from build123d import *

# Parameters (mm, degrees)
SKETCH_1_R          = 13
EXTRUDE_2_DEPTH     = 10
CUT_EXTRUDE_1_DEPTH = 21.928449536
SKETCH_3_R          = 7.5
CUT_EXTRUDE_2_DEPTH = 4
CUT_EXTRUDE_2_DRAFT = 6
SKETCH_4_R          = 7.5
CUT_EXTRUDE_3_DEPTH = 4
CUT_EXTRUDE_3_DRAFT = 6
SKETCH_5_R          = 4
EXTRUDE_3_DEPTH     = 30
CHAMFER_1_SIZE      = 1


with BuildPart() as part:
    # Эскиз1 → Бобышка-Вытянуть2 (new body)
    with BuildSketch(Plane.XY):
        Circle(SKETCH_1_R)
    extrude(amount=-EXTRUDE_2_DEPTH)

    # Эскиз2 → Вырез-Вытянуть1 (cut, through all)
    with BuildSketch(Plane.XY):
        with BuildLine():
            ThreePointArc((1.252557909, 8.912412619), (0, 9), (-1.252557909, 8.912412619))
            ThreePointArc((-1.252557909, 8.912412619), (-1.684886314, 10.969320472), (-2.924363706, 12.666810842))
            ThreePointArc((-2.924363706, 12.666810842), (0, 13), (2.924363706, 12.666810842))
            ThreePointArc((2.924363706, 12.666810842), (1.684886314, 10.969320472), (1.252557909, 8.912412619))
        make_face()
        with BuildLine():
            ThreePointArc((9.308326268, 9.074968986), (7.028330627, 10.936295927), (4.388063669, 12.237029756))
            ThreePointArc((4.388063669, 12.237029756), (4.513045823, 10.138897913), (3.764695278, 8.174782533))
            ThreePointArc((3.764695278, 8.174782533), (4.865767357, 7.571281795), (5.872132809, 6.82041467))
            ThreePointArc((5.872132809, 6.82041467), (7.34787895, 8.317061286), (9.308326268, 9.074968986))
        make_face()
        with BuildLine():
            ThreePointArc((12.736961008, 2.601888597), (11.82521594, 5.400395169), (10.307311834, 7.922078184))
            ThreePointArc((10.307311834, 7.922078184), (9.278117798, 6.089446906), (7.586684314, 4.841716754))
            ThreePointArc((7.586684314, 4.841716754), (8.186687958, 3.738735117), (8.627347034, 2.562983254))
            ThreePointArc((8.627347034, 2.562983254), (10.677971938, 3.024193907), (12.736961008, 2.601888597))
        make_face()
        with BuildLine():
            ThreePointArc((12.121700624, -4.697273037), (12.867678744, -1.850092898), (12.95406132, 1.091922764))
            ThreePointArc((12.95406132, 1.091922764), (11.097452929, 0.106639531), (8.999954685, -0.028559885))
            ThreePointArc((8.999954685, -0.028559885), (8.908392977, -1.280833544), (8.643439533, -2.508177236))
            ThreePointArc((8.643439533, -2.508177236), (10.617884283, -3.228833669), (12.121700624, -4.697273037))
        make_face()
        with BuildLine():
            ThreePointArc((7.657885939, -10.505083671), (9.824744467, -8.513189541), (11.487987866, -6.084910418))
            ThreePointArc((11.487987866, -6.084910418), (9.393425165, -5.910025141), (7.555803034, -4.889768962))
            ThreePointArc((7.555803034, -4.889768962), (6.801746169, -5.893746606), (5.915301052, -6.783009175))
            ThreePointArc((5.915301052, -6.783009175), (7.186693389, -8.456729369), (7.657885939, -10.505083671))
        make_face()
        with BuildLine():
            ThreePointArc((0.762746577, -12.977604465), (3.662523239, -12.473408657), (6.374559434, -11.329827537))
            ThreePointArc((6.374559434, -11.329827537), (4.707051283, -10.050298589), (3.712737307, -8.198510943))
            ThreePointArc((3.712737307, -8.198510943), (2.535593012, -8.635436763), (1.309096282, -8.904283628))
            ThreePointArc((1.309096282, -8.904283628), (1.473778124, -10.999673247), (0.762746577, -12.977604465))
        make_face()
        with BuildLine():
            ThreePointArc((-6.374559434, -11.329827537), (-3.662523239, -12.473408657), (-0.762746577, -12.977604465))
            ThreePointArc((-0.762746577, -12.977604465), (-1.473778124, -10.999673247), (-1.309096282, -8.904283628))
            ThreePointArc((-1.309096282, -8.904283628), (-2.535593012, -8.635436763), (-3.712737307, -8.198510943))
            ThreePointArc((-3.712737307, -8.198510943), (-4.707051283, -10.050298589), (-6.374559434, -11.329827537))
        make_face()
        with BuildLine():
            ThreePointArc((-11.487987866, -6.084910418), (-9.824744467, -8.513189541), (-7.657885939, -10.505083671))
            ThreePointArc((-7.657885939, -10.505083671), (-7.186693389, -8.456729369), (-5.915301052, -6.783009175))
            ThreePointArc((-5.915301052, -6.783009175), (-6.801746169, -5.893746606), (-7.555803034, -4.889768962))
            ThreePointArc((-7.555803034, -4.889768962), (-9.393425165, -5.910025141), (-11.487987866, -6.084910418))
        make_face()
        with BuildLine():
            ThreePointArc((-12.95406132, 1.091922764), (-12.867678744, -1.850092898), (-12.121700624, -4.697273037))
            ThreePointArc((-12.121700624, -4.697273037), (-10.617884283, -3.228833669), (-8.643439533, -2.508177236))
            ThreePointArc((-8.643439533, -2.508177236), (-8.908392977, -1.280833544), (-8.999954685, -0.028559885))
            ThreePointArc((-8.999954685, -0.028559885), (-11.097452929, 0.106639531), (-12.95406132, 1.091922764))
        make_face()
        with BuildLine():
            ThreePointArc((-10.307311834, 7.922078184), (-11.82521594, 5.400395169), (-12.736961008, 2.601888597))
            ThreePointArc((-12.736961008, 2.601888597), (-10.677971938, 3.024193907), (-8.627347034, 2.562983254))
            ThreePointArc((-8.627347034, 2.562983254), (-8.186687958, 3.738735117), (-7.586684314, 4.841716754))
            ThreePointArc((-7.586684314, 4.841716754), (-9.278117798, 6.089446906), (-10.307311834, 7.922078184))
        make_face()
        with BuildLine():
            ThreePointArc((-4.388063669, 12.237029756), (-7.028330627, 10.936295927), (-9.308326268, 9.074968986))
            ThreePointArc((-9.308326268, 9.074968986), (-7.34787895, 8.317061286), (-5.872132809, 6.82041467))
            ThreePointArc((-5.872132809, 6.82041467), (-4.865767357, 7.571281795), (-3.764695278, 8.174782533))
            ThreePointArc((-3.764695278, 8.174782533), (-4.513045823, 10.138897913), (-4.388063669, 12.237029756))
        make_face()
    extrude(amount=-CUT_EXTRUDE_1_DEPTH, mode=Mode.SUBTRACT)


with BuildPart() as cut_extrude_2_tool:
    # Эскиз3 → Вырез-Вытянуть2 (with draft: the straight prism first)
    with BuildSketch(Plane.XY):
        Circle(SKETCH_3_R)
    extrude(amount=-CUT_EXTRUDE_2_DEPTH)
    # Вырез-Вытянуть2: the draft: its side faces are tilted about the plane it starts from
    cut_extrude_2_sides = [cut_extrude_2_tool.faces().sort_by_distance(p)[0] for p in [
        (-7.5, 0, -2),
    ]]
    draft(cut_extrude_2_sides, Plane.XY, CUT_EXTRUDE_2_DRAFT)


with BuildPart() as part_1:
    add(part.part)

    # Вырез-Вытянуть2: cut by cut_extrude_2_tool
    add(cut_extrude_2_tool.part, mode=Mode.SUBTRACT)


with BuildPart() as cut_extrude_3_tool:
    # Эскиз4 → Вырез-Вытянуть3 (with draft: the straight prism first)
    with BuildSketch(Plane(origin=(0, 0, -10), x_dir=(-1, 0, 0), z_dir=(0, 0, -1))):
        Circle(SKETCH_4_R)
    extrude(amount=-CUT_EXTRUDE_3_DEPTH)
    # Вырез-Вытянуть3: the draft: its side faces are tilted about the plane it starts from
    cut_extrude_3_sides = [cut_extrude_3_tool.faces().sort_by_distance(p)[0] for p in [
        (7.5, 0, -8),
    ]]
    draft(cut_extrude_3_sides, Plane(origin=(0, 0, -10), x_dir=(-1, 0, 0), z_dir=(0, 0, -1)), CUT_EXTRUDE_3_DRAFT)


with BuildPart() as part_2:
    add(part_1.part)

    # Вырез-Вытянуть3: cut by cut_extrude_3_tool
    add(cut_extrude_3_tool.part, mode=Mode.SUBTRACT)

    # Эскиз5 → Бобышка-Вытянуть3 (add)
    with BuildSketch(Plane.XY.offset(-4)):
        Circle(SKETCH_5_R)
    extrude(amount=EXTRUDE_3_DEPTH)

    # Фаска1
    chamfer_1_edges = [part_2.edges().sort_by_distance(p)[0] for p in [
        (-4, 0, 26),
    ]]
    chamfer(chamfer_1_edges, length=CHAMFER_1_SIZE)


solid = part_2.part
Could you check a few things on this model? Use its own coordinates, in mm. A direction names the side the tool comes from. Give positions to 0.01 mm unless a question says otherwise; leave off trailing zeros. Write each loop counter-clockwise with the first axis right and the second up, starting at its lowest first coordinate (ties: lowest second). Pieces come first, ordered by that corner, then holes. Notation, with made-up numbers: (-12, 17) -> (-1, 17) arc R19 cw to (-1, 21) -> close; hole circle Ø11 at (76, 39.5). An arc over 180 degrees is marked (long way). Answer as a JSON object with one key per item and string values.
Q1. Suppose I cut it at B-B on z = 20.5. Write out the boundary of the cut face in (x, y), then the cut area to 3 significant figures.
Taken from the geometry:
{"outline": "circle Ø8 at (0, 0)", "area": "50.3 mm²"}
Q2. We'd pull the mould along Y, two halves only. Please class faces 4 (the cylindrical face through (-10.643, -3.245, -4.93)), 5 (the cylindrical face through (12.87, 1.84, -4.93)), 6 (the flat face through (-5, -6, 0)): released by +Y, released by -Y, zero draft, split by the parting line, or undercut.
Taken from the geometry:
{"face 4": "undercut", "face 5": "released by +Y", "face 6": "zero draft"}
Q3. Will these pins go through, and if not, where does the flat tip stop? pin 1 Ø10 at (x, y) = (-10.5, -6.5) entering from +Z; pin 2 Ø6 at (x, z) = (9, 2.5) entering from +Y; pin 3 Ø2 at (y, z) = (-5.5, 15.5) entering from -X; pin 4 Ø5 at (x, z) = (0, -4) entering from +Y.
Taken from the geometry:
{"pin 1": "stops at z = 0", "pin 2": "stops at y = 9.07", "pin 3": "passes through", "pin 4": "stops at y = 12.24"}
Q4. Please list where these lines run through material, in increasing order: L1, parallel to Y at x = 0.5, z = -8; L2, parallel to Z at x = -2.75, y = 3.75; L3, parallel to Z at x = 1.75, y = -2.25.
Taken from the geometry:
{"L1": "y = -12.99 to -7.69, 7.69 to 8.99", "L2": "z = -6 to -4", "L3": "z = -6 to 26"}
Q5. Which directions (+Z, -Z, +X, -X, +Y, -Y) give clear straight access to the entire face, cutting with the end or side of a thin tool? Please do faces 1 (the flat face through (-5, -6, -10)), 2 (the cylindrical face through (-0.867, -3.905, 10.297)), 3 (the conical face through (-1.651, -7.433, -1.083)).
Taken from the geometry:
{"face 1": "-Z, +X, -X, +Y, -Y", "face 2": "+Z", "face 3": "none"}
Q6. Suppose I cut it at A-A on x = 0. Write out the boundary of the cut face in (y, z), then the cut area to 3 significant figures.
Taken from the geometry:
{"outline": "(-13, -10) -> (-7.5, -10) -> (-7.92, -6) -> (7.92, -6) -> (7.5, -10) -> (9, -10) -> (9, 0) -> (7.5, 0) -> (7.92, -4) -> (4, -4) -> (4, 25) -> (3, 26) -> (-3, 26) -> (-4, 25) -> (-4, -4) -> (-7.92, -4) -> (-7.5, 0) -> (-13, 0) -> close", "area": "336 mm²"}
